Can you work these out from the model? Positions are in its coordinate system, mm. A direction names the side the tool comes from. Coordinates: 2 decimals unless noted, no trailing zeros. Loops run counter-clockwise (first coordinate to the right, second up) from the corner with the lowest first, then second, coordinate; pieces in that order, holes last. Notation, with made-up numbers: M 9,39.5 L 47,39.5 A9 ccw 47,55.5 Z; hole C -36,54.5 d3. An arc over 180 degrees is marked long. Answer as a JSON object with one key per item and string values. Group by question number.
Item 1: If I drill on line 1 (X direction, y = 54, z = 5.35); line 2 (X direction, y = 6, z = 3.55); line 3 (Y direction, x = -3.5, z = 1.45), over which ranges is the centre line in solid material (lowest first)?
Item 2: I'm going to push flat-ended pins straight in: pin 1 Ø3.5 at (x, y) = (0, 54) entering from +Z; pin 2 Ø2.5 at (x, y) = (0, -54) entering from +Z; pin 3 Ø3.5 at (x, y) = (-0.5, 54) entering from +Z; pin 4 Ø2 at (x, z) = (-4.5, 2) entering from +Y. Where does each tip first touch, or does it pass through?
Item 3: Suppose I cut it at D-D (x = -8). Write out the boundary of the cut face in (y, z).
Item 4: We'd pull the mould along Y, two halves only. Please class faces 3 (the flat face through (-5, -7, 4)), 4 (the flat face through (0, -25, 2)), 5 (the flat face through (0, 47.95, 5)): +Y half, -Y half, draft (parallel to the pull), parting line (faces both ways), or undercut.
Item 5: Suppose I cut it at C-C (x = 4.75). Write out the boundary of the cut face in (y, z), then the cut area to 3 significant figures.
Item 6: Which directions (+Z, -Z, +X, -X, +Y, -Y) give clear straight access to the entire face, cutting with the end or side of a thin tool? Please do faces 1 (the cylindrical face through (0, -64, 2)), 2 (the flat face through (0, -10, 2)).
Item 7: Suppose I cut it at B-B (x = 0). Count the separate pieces of the cut face and the enclosed holes in it, then the cut area to 3 significant figures.
Item 8: Suppose I cut it at A-A (z = 2.8). Write out the boundary of the cut face in (x, y), then the cut area to 3 significant figures.
```python
from build123d import *

# Parameters (mm, degrees)
CROQUIS1_R              = 2.1
SALIENTE_EXTRUIR1_DEPTH = 4
CROQUIS1_6_R            = 2.1
SALIENTE_EXTRUIR3_DEPTH = 6


with BuildPart() as part:
    # Croquis1 → Saliente-Extruir1 (new body)
    with BuildSketch(Plane.XY):
        with BuildLine():
            ThreePointArc((10, 54), (0, 64), (-10, 54))
            Line((-10, 54), (-10, -54))
            ThreePointArc((-10, -54), (0, -64), (10, -54))
            Line((10, -54), (10, 54))
        make_face()
        with BuildLine():
            Line((6, 38), (6, 22))
            Line((6, 22), (-6, 34))
            Line((-6, 34), (-6, 38))
            ThreePointArc((-6, 38), (0, 44), (6, 38))
        make_face(mode=Mode.SUBTRACT)
        Polygon((6, 16), (6, -16), (-6, -4), (-6, 4), align=None, mode=Mode.SUBTRACT)
        with BuildLine():
            Line((6, -22), (6, -38))
            ThreePointArc((6, -38), (0, -44), (-6, -38))
            Line((-6, -38), (-6, -34))
            Line((-6, -34), (6, -22))
        make_face(mode=Mode.SUBTRACT)
        Polygon((-6, -31), (-6, -7), (6, -19), align=None, mode=Mode.SUBTRACT)
        Polygon((-6, 7), (-6, 31), (6, 19), align=None, mode=Mode.SUBTRACT)
        with Locations((0, -54)):
            Circle(CROQUIS1_R, mode=Mode.SUBTRACT)
    extrude(amount=SALIENTE_EXTRUIR1_DEPTH)

    # Croquis1_6 → Saliente-Extruir3 (add)
    with BuildSketch(Plane.XY):
        with BuildLine():
            Line((10, 47.95), (10, 54))
            ThreePointArc((10, 54), (0, 64), (-10, 54))
            Line((-10, 54), (-10, 47.95))
            Line((-10, 47.95), (10, 47.95))
        make_face()
        with Locations((0, 54)):
            Circle(CROQUIS1_6_R, mode=Mode.SUBTRACT)
    extrude(amount=SALIENTE_EXTRUIR3_DEPTH)


solid = part.part
```
From the geometry:
{
 "1": {"line 1": "-10 to -2.1, 2.1 to 10", "line 2": "-10 to -4, 6 to 10", "line 3": "-63.37 to -42.87, -31.5 to -28.5, -9.5 to -6.5, 6.5 to 9.5, 28.5 to 31.5, 42.87 to 63.37"},
 "2": {"pin 1": "z = 4", "pin 2": "through", "pin 3": "z = 6", "pin 4": "y = 63.37"},
 "3": {"outline": "M -60,0 L 60,0 L 60,6 L 47.95,6 L 47.95,4 L -60,4 Z"},
 "4": {"face 3": "draft", "face 4": "undercut", "face 5": "-Y half"},
 "5": {"outline": "M -62.8,0 L -41.67,0 L -41.67,4 L -62.8,4 Z; M -23.25,0 L -20.25,0 L -20.25,4 L -23.25,4 Z; M -17.75,0 L -14.75,0 L -14.75,4 L -17.75,4 Z; M 14.75,0 L 17.75,0 L 17.75,4 L 14.75,4 Z; M 20.25,0 L 23.25,0 L 23.25,4 L 20.25,4 Z; M 41.67,0 L 62.8,0 L 62.8,6 L 47.95,6 L 47.95,4 L 41.67,4 Z", "area": "247 mm2"},
 "6": {"face 1": "+Z, -Z, -Y", "face 2": "+Z, -Z"},
 "7": {"separate pieces": "7", "enclosed holes": "0", "area": "215 mm2"},
 "8": {"outline": "M -10,-54 A10 ccw 10,-54 L 10,54 A10 ccw -10,54 Z; hole M -6,-38 A6 ccw 6,-38 L 6,-22 L -6,-34 Z; hole M -6,-31 L 6,-19 L -6,-7 Z; hole M -6,-4 L 6,-16 L 6,16 L -6,4 Z; hole M -6,7 L 6,19 L -6,31 Z; hole M -6,34 L 6,22 L 6,38 A6 ccw -6,38 Z; hole C 0,-54 d4.2", "area": "1,580 mm2"}
}
